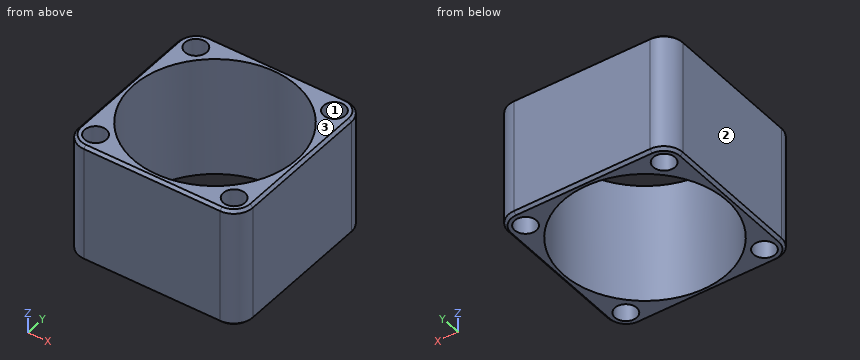
Autodesk Inventor part; units mm, degrees
ref_plane "YZ Plane" through (0, 0, 0) normal (1, 0, 0) x (0, 1, 0)
ref_plane "XZ Plane" through (0, 0, 0) normal (0, 1, 0) x (-1, 0, 0)
ref_plane "XY Plane" through (0, 0, 0) normal (0, 0, 1) x (1, 0, 0)
sketch "Sketch1" plane through (0, 0, 0) normal (0, 0, 1) x (1, 0, 0)
  circle A0 centre (0, 0) radius 11
  circle A1 centre (0, 0) radius 9 construction
  line L0 (0, 0) -> (0, 11) construction
  line L1 (0, 0) -> (-6.364, 6.364) construction
  circle A2 centre (-6.364, 6.364) radius 1
  circle A3 centre (0, 0) radius 7.5
  circle A4 centre (-6.364, -6.364) radius 1
  circle A5 centre (6.364, -6.364) radius 1
  circle A6 centre (6.364, 6.364) radius 1
  dimension "d0" = 22
  dimension "d1" = 18
  dimension "d2" = 45
  dimension "d3" = 2
  dimension "d4" = 15
  dimension "d7" = 360
extrude "Extrusion1" add sketch "Sketch1" along normal blind 11
chamfer "Chamfer1" [suppressed]
chamfer "Chamfer2" [suppressed]
sketch "Sketch2" plane through (0, 0, 11) normal (0, 0, 1) x (1, 0, 0)
  line L0 (8, -8) -> (-8, -8)
  line L1 (-8, -8) -> (-8, 8)
  line L2 (-8, 8) -> (8, 8)
  line L3 (8, 8) -> (8, -8)
  line L4 (8, -8) -> (-8, 8) construction
  line L5 (-8, -8) -> (8, 8) construction
  circle A0 centre (0, 0) radius 15
  arc A1 (-6.25, 8) -> (-8, 6.25) centre (-6.25, 6.25) ccw
  arc A2 (-8, -6.25) -> (-6.25, -8) centre (-6.25, -6.25) ccw
  arc A3 (6.25, -8) -> (8, -6.25) centre (6.25, -6.25) ccw
  arc A4 (8, 6.25) -> (6.25, 8) centre (6.25, 6.25) ccw
  point P0 (8, 6.25)
  point P1 (8, -6.25)
  point P2 (6.25, -8)
  point P3 (-6.25, -8)
  point P4 (-8, -6.25)
  point P5 (6.25, 8)
  dimension "d11" = 16
  dimension "d12" = 16
  dimension "d13" = 30
  dimension "d14" = 3.5
  dimension "d17" = 360
extrude "Extrusion2" cut sketch "Sketch2" against normal through all contours L0 A3 L3 | L0 L1 A2 | A4 L2 L3 | L1 L2 A1 | A0
chamfer "Chamfer3" distance 0.25 angle 45 16 edges at (8, 0, 11) (7.4874, 7.4874, 11) (0, 8, 11) (-7.4874, 7.4874, 11) (-8, 0, 11) (-7.4874, -7.4874, 11) (0, -8, 11) (7.4874, -7.4874, 11) (8, 0, 0) (7.4874, -7.4874, 0) (0, -8, 0) (-7.4874, -7.4874, 0) (-8, 0, 0) (-7.4874, 7.4874, 0) (0, 8, 0) (7.4874, 7.4874, 0)
properties part number "AL Ring" material "Aluminum 6061"
Could you check a few things on this model? Use its own coordinates, in mm. Face numbers are marked on the shaded views. Give positions to 0.01 mm unless a question says otherwise; leave off trailing zeros. Loops run counter-clockwise (first coordinate to the right, second up) from the corner with the lowest first, then second, coordinate; pieces in that order, holes last. Notation, with made-up numbers: (32, 34) -> (63, 34) arc R9 cw to (63, 47) -> close; hole circle Ø9 at (84, 44). An arc over 180 degrees is marked (long way). Put each result on its own line as item: value.
(1) I'm going to push a flat-ended pin straight in: pin 1 Ø1.8 at (x, y) = (6.364, 6.364) entering from -Z. Where does the tip first touch, or does it pass through?
Computed:
pin 1: through
(2) Imagine slicing it at D-D on x = 6.5. State how many separate pieces and enclosed holes the cut face has, plus the area to 3 significant figures.
Computed:
separate pieces: 4
enclosed holes: 0
area: 49.6 mm^2
(3) Please list where these lines run through material, in increasing order: probe 1 along X at (y, z) = (6.75, 10); probe 2 along X at (y, z) = (-5.75, 9); probe 3 along X at (y, z) = (1.25, 3.75). Write a range as [from, to].
Computed:
probe 1: [-7.93, -7.29], [-5.44, -3.27], [3.27, 5.44], [7.29, 7.93]
probe 2: [-8, -7.15], [-5.57, -4.82], [4.82, 5.57], [7.15, 8]
probe 3: [-8, -7.4], [7.4, 8]
(4) Imagine slicing it at A-A on y = 0. Write out the boundary of the cut face in (x, z).
Computed:
outline: (-8, 0.25) -> (-7.75, 0) -> (-7.5, 0) -> (-7.5, 11) -> (-7.75, 11) -> (-8, 10.75) -> close; (7.5, 0) -> (7.75, 0) -> (8, 0.25) -> (8, 10.75) -> (7.75, 11) -> (7.5, 11) -> close
(5) Imagine slicing it at C-C on z = 1.75. Write out the boundary of the cut face in (x, y), plus the area to 3 significant figures.
Computed:
outline: (-8, -6.25) arc R1.75 ccw to (-6.25, -8) -> (6.25, -8) arc R1.75 ccw to (8, -6.25) -> (8, 6.25) arc R1.75 ccw to (6.25, 8) -> (-6.25, 8) arc R1.75 ccw to (-8, 6.25) -> close; hole circle Ø15 at (0, 0); hole circle Ø2 at (-6.36, -6.36); hole circle Ø2 at (-6.36, 6.36); hole circle Ø2 at (6.36, -6.36); hole circle Ø2 at (6.36, 6.36)
area: 64.1 mm^2
(6) Thinking about a two-plate mould opening in X: for the marked faces 1, 2 and 3, which applies, pulls with the +X half, pulls with the -X half, needs draft (parallel to the pull), parting line crosses it, or undercut?
Computed:
face 1: undercut
face 2: pulls with the -X half
face 3: needs draft
